Check sheet for the modelled part. Datum: model origin and axes. Units: mm. Coordinates: 2 decimals unless noted, no trailing zeros. Write each loop counter-clockwise with the first axis right and the second up, starting at its lowest first coordinate (ties: lowest second). Pieces come first, ordered by that corner, then holes. Notation, with made-up numbers: (15.25, -17) -> (54.25, -17) arc R13 cw to (54.25, -4) -> close; hole circle Ø3 at (63.25, 31). An arc over 180 degrees is marked (long way). Put each result on its own line as item: value.
Autodesk Inventor part; units mm, degrees
ref_plane "YZ Plane" through (0, 0, 0) normal (1, 0, 0) x (0, 1, 0)
ref_plane "XZ Plane" through (0, 0, 0) normal (0, 1, 0) x (-1, 0, 0)
ref_plane "XY Plane" through (0, 0, 0) normal (0, 0, 1) x (1, 0, 0)
sketch "Sketch1" plane through (0, 0, 0) normal (0, 1, 0) x (-1, 0, 0)
  circle A0 centre (0, 0) radius 84.75
  dimension "d0" = 169.5
extrude "Extrusion1" add sketch "Sketch1" along normal blind 15
sketch "Sketch2" plane through (0, 0, 0) normal (0, -1, 0) x (1, 0, 0)
  circle A0 centre (0, 0) radius 76
  circle A1 centre (0, 76) radius 4
  circle A2 centre (0, -76) radius 4
  circle A3 centre (0, 76) radius 2.25
  circle A4 centre (0, -76) radius 2.25
  dimension "d3" = 152
  dimension "d4" = 8
  dimension "d5" = 8
  dimension "d6" = 4.5
  dimension "d7" = 4.5
extrude "Extrusion2" cut sketch "Sketch2" against normal through all contours A3 A0 | A0 A3 | A4 A0 | A0 A4
extrude "Extrusion3" cut sketch "Sketch2" against normal blind 12 contours A1 A0 A3 | A0 A3 A1 | A2 A0 A4 | A0 A4 A2 | A3 A0 | A0 A3 | A4 A0 | A0 A4
sketch "Sketch3" plane through (0, 0, 0) normal (0, -1, 0) x (1, 0, 0)
  circle A0 centre (0, 0) radius 84.75
  circle A1 centre (0, 0) radius 20
  circle A2 centre (0, -20) radius 4
  circle A3 centre (20, 0) radius 4
  circle A4 centre (0, 20) radius 4
  circle A5 centre (-20, 0) radius 4
  line L0 (55, 55) -> (-55, 55)
  line L1 (-55, 55) -> (-55, -55)
  line L2 (-55, -55) -> (55, -55)
  line L3 (55, -55) -> (55, 55)
  line L4 (55, 55) -> (-55, -55) construction
  line L5 (-55, 55) -> (55, -55) construction
  circle A6 centre (0, 0) radius 55
  circle A7 centre (-38.8909, -38.8909) radius 4
  circle A8 centre (38.8909, -38.8909) radius 4
  circle A9 centre (38.8909, 38.8909) radius 4
  circle A10 centre (-38.8909, 38.8909) radius 4
  dimension "d12" = 40
  dimension "d13" = 8
  dimension "d16" = 360
  dimension "d21" = 110
  dimension "d22" = 110
  dimension "d23" = 110
  dimension "d24" = 8
  dimension "d25" = 8
  dimension "d26" = 8
  dimension "d27" = 8
hole "Hole1" at (38.8909, 0, -38.8909) at (38.8909, 0, 38.8909) at (-38.8909, 0, 38.8909) at (-38.8909, 0, -38.8909) direction (0, 1, 0) diameter 6.647 depth 12 tip angle 118
properties part number "Modified Substrate Plate Top"
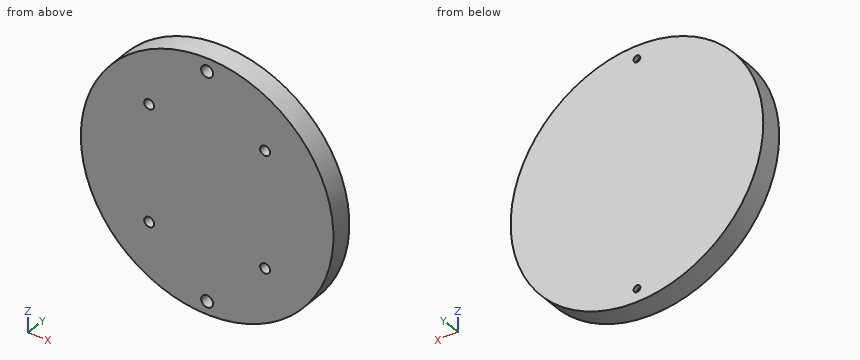
Q1. Cross-section at D-D (z = -16.5). Record the cut outline in (x, y).
Recorded:
outline: (-83.13, 0) -> (83.13, 0) -> (83.13, 15) -> (-83.13, 15) -> close
Q2. Cross-section at A-A (x = 0). Record the cut outline in (y, z).
Recorded:
outline: (0, -84.75) -> (15, -84.75) -> (15, -78.25) -> (12, -78.25) -> (12, -80) -> (0, -80) -> close; (0, -72) -> (12, -72) -> (12, -73.75) -> (15, -73.75) -> (15, 73.75) -> (12, 73.75) -> (12, 72) -> (0, 72) -> close; (0, 80) -> (12, 80) -> (12, 78.25) -> (15, 78.25) -> (15, 84.75) -> (0, 84.75) -> close
Q3. Cross-section at B-B (z = 76). Record the cut outline in (x, y).
Recorded:
outline: (-37.5, 0) -> (-4, 0) -> (-4, 12) -> (-2.25, 12) -> (-2.25, 15) -> (-37.5, 15) -> close; (2.25, 12) -> (4, 12) -> (4, 0) -> (37.5, 0) -> (37.5, 15) -> (2.25, 15) -> close
Q4. Material ranges on line 1 along Z through (x, y) = (0, 12.6); line 2 along Z through (x, y) = (0, 8.25); line 3 along X through (y, z) = (8.25, 37.5), recorded low to high.
Recorded:
line 1: z = -84.75 to -78.25, -73.75 to 73.75, 78.25 to 84.75
line 2: z = -84.75 to -80, -72 to 72, 80 to 84.75
line 3: x = -76 to -41.91, -35.87 to 35.87, 41.91 to 76
Q5. Cross-section at C-C (x = 22). Record the cut outline in (y, z), plus the area to 3 significant figures.
Recorded:
outline: (0, -81.84) -> (15, -81.84) -> (15, 81.84) -> (0, 81.84) -> close
area: 2,460 mm2
Q6. Depth check by flat-ended pin: P1, Ø4, axis at x = 1.5, z = -78, coming from the -Y side; P2, Ø8, axis at y = 5.5, z = -35, coming from the -X side; P3, Ø1.5, axis at y = 1.5, z = -27.5, coming from the -X side; P4, Ø1.5, axis at x = -54.5, y = 12, coming from the -Z side. Enter the tip coordinate at first touch or a pass-through.
Recorded:
P1: stops at y = 0
P2: stops at x = -78.88
P3: stops at x = -80.42
P4: stops at z = -65.52
